Can you work these out from the drawing? Everything is in mm from the part's minimum corner. A direction names the side the tool comes from. Round coordinates to 2 decimals unless told otherwise and drop trailing zeros. Write each loop counter-clockwise with the first axis right and the second up, starting at its lowest first coordinate (ties: lowest second). Pieces come first, ordered by that corner, then holes. Notation, with made-up numbers: (11.5, 44.25) - (53.5, 44.25) arc R29 ccw to (53.5, 68.25) - close; hole circle Ø11 at (60.25, -34.5). An arc over 180 degrees is marked (long way). One line per item, written item: value. Start each with the question number.
(1) On a 3-axis mill with a long thin cutter (end or side, diameter ignored), from which of +Z, -Z, +X, -X, +Y, -Y can I reach the whole of each face in a straight line? I mean the marked faces 1 and 2. Say none if no direction works.
(2) I want a section at B-B on x = 15. List the corners of the cut face in (y, z) for me, plus the area to 3 significant figures.
(3) Thinking about a two-plate mould opening in Y: for the marked faces 3, 4 and 5, which applies, +Y half, -Y half, draft (parallel to the pull), parting line (faces both ways), or undercut?
(4) I want a section at A-A on y = 54. List the corners of the cut face in (x, z) for me.
(5) I want a section at D-D on x = 35. List the corners of the cut face in (y, z) for me, plus the area to 3 significant figures.
(6) I'm going to push flat-ended pins straight in: pin 1 Ø8 at (y, z) = (60.02, 5.25) entering from -X; pin 2 Ø11 at (x, y) = (20, 48.5) entering from -Z. Where does each tip first touch, or does it pass through?
(7) If I drill on L1, parallel to Y at x = 15, z = 88; L2, parallel to Y at x = 11, z = 59.5; L3, parallel to X at y = 14, z = 84, over which ranges is the centre line in solid material (lowest first)? Write a range as from..to.
(8) I want a section at C-C on z = 54.75. List the corners of the cut face in (x, y) for me, plus the area to 3 significant figures.
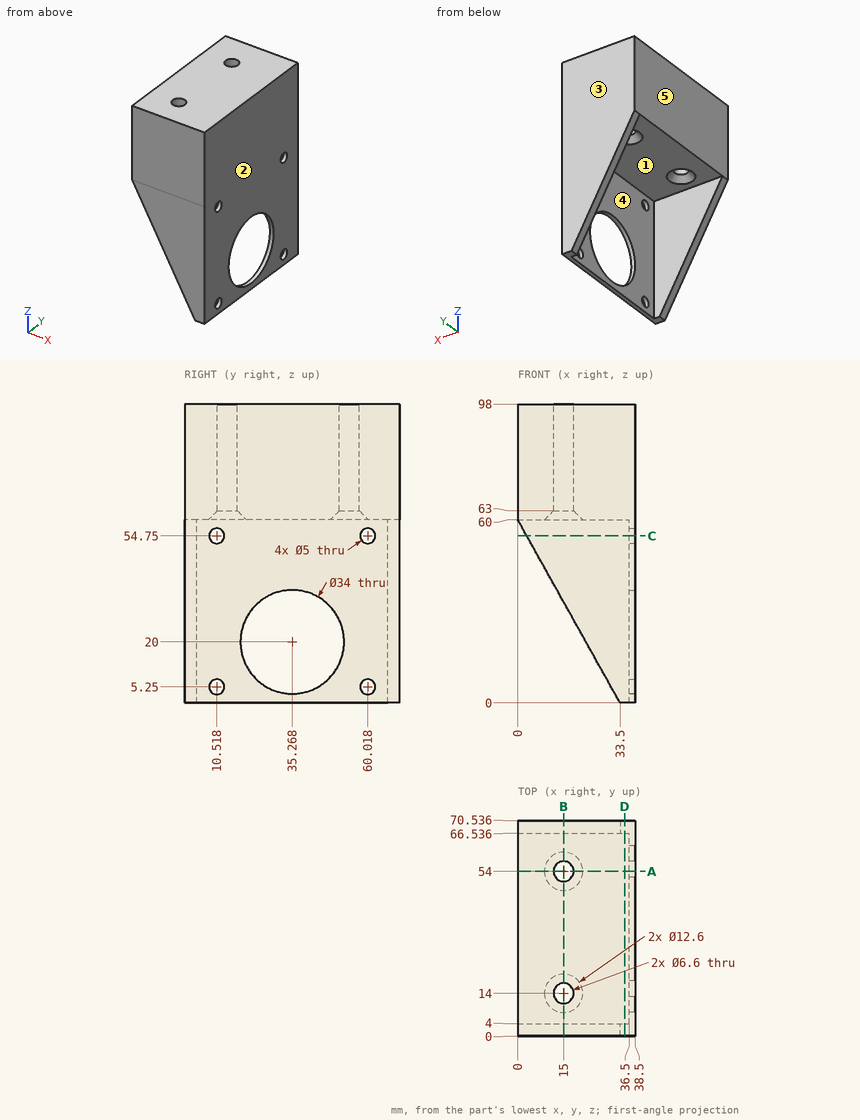
Established:
1. face 1: -Z, -X
1. face 2: +Z, -Z, +X, +Y, -Y
2. outline: (0, 33.13) - (4, 33.13) - (4, 60) - (7.7, 60) - (10.7, 63) - (10.7, 98) - (0, 98) - close; (17.3, 63) - (20.3, 60) - (47.7, 60) - (50.7, 63) - (50.7, 98) - (17.3, 98) - close; (57.3, 63) - (60.3, 60) - (66.54, 60) - (66.54, 33.13) - (70.54, 33.13) - (70.54, 98) - (57.3, 98) - close
2. area: 2,380 mm2
3. face 3: +Y half
3. face 4: undercut
3. face 5: draft
4. outline: (0, 60) - (8.7, 60) - (11.7, 63) - (11.7, 98) - (0, 98) - close; (18.3, 63) - (21.3, 60) - (36.5, 60) - (36.5, 0) - (38.5, 0) - (38.5, 98) - (18.3, 98) - close
5. outline: (0, 0) - (4, 0) - (4, 60) - (66.54, 60) - (66.54, 0) - (70.54, 0) - (70.54, 98) - (0, 98) - close
5. area: 3,160 mm2
6. pin 1: x = 36.5
6. pin 2: z = 60
7. L1: 0..10.7, 17.3..50.7, 57.3..70.54
7. L2: 0..4, 66.54..70.54
7. L3: 0..11.7, 18.3..38.5
8. outline: (2.93, 0) - (38.5, 0) - (38.5, 8.02) - (36.5, 8.02) - (36.5, 4) - (2.93, 4) - close; (2.93, 66.54) - (36.5, 66.54) - (36.5, 62.52) - (38.5, 62.52) - (38.5, 70.54) - (2.93, 70.54) - close; (36.5, 13.02) - (38.5, 13.02) - (38.5, 57.52) - (36.5, 57.52) - close
8. area: 390 mm2
